```python
from build123d import *

# Parameters (mm, degrees)
SKETCH_R    = 4.3
PAD_DEPTH   = 20
FILLET_R    = 2.5
FILLET001_R = 5


with BuildPart() as part:
    # Sketch → Pad (new body)
    with BuildSketch(Plane.XY):
        with BuildLine():
            ThreePointArc((7, 0), (0, 7), (-7, 0))
            ThreePointArc((-10.818791, -6.235375), (-8.030558, -3.655922), (-7, 0))
            Line((-10.818791, -6.235375), (10.818791, -6.235375))
            ThreePointArc((7, 0), (8.030558, -3.655922), (10.818791, -6.235375))
        make_face()
        Circle(SKETCH_R, mode=Mode.SUBTRACT)
    extrude(amount=PAD_DEPTH)

    # Fillet
    fillet_edges = [part.edges().sort_by_distance(p)[0] for p in [
        (0, 7, 20),
        (8.030558, -3.655922, 20),
        (-8.030558, -3.655922, 20),
    ]]
    fillet(fillet_edges, radius=FILLET_R)

    # Fillet001
    fillet001_edges = [part.edges().sort_by_distance(p)[0] for p in [
        (0, 7, 0),
        (-8.030558, -3.655922, 0),
        (8.030558, -3.655922, 0),
    ]]
    fillet(fillet001_edges, radius=FILLET001_R)


solid = part.part
```
Check sheet for the modelled part. Datum: model origin and axes. Units: mm. Coordinates: 2 decimals unless noted, no trailing zeros. Write each loop counter-clockwise with the first axis right and the second up, starting at its lowest first coordinate (ties: lowest second). Pieces come first, ordered by that corner, then holes. Notation, with made-up numbers: (69, 49) - (107, 49) arc R11 cw to (107, 66) - close; hole circle Ø3 at (-26, 22.25). An arc over 180 degrees is marked (long way). One line per question, with ' | ' between items.
Item 1: Thickness scan on line 1 (X direction, y = 0, z = 12); line 2 (Y direction, x = 0, z = 8); line 3 (Y direction, x = 7.25, z = 2). Record the ranges inside material, lowest first. Write a range as [from, to].
Determined:
line 1: x = [-7, -4.3], [4.3, 7] | line 2: y = [-6.24, -4.3], [4.3, 7] | line 3: y = [-6.24, -4.29]
Item 2: Gauge pin test, flat ends, axial feed: P1, Ø10, axis at x = 4.5, z = 6.5, coming from the +Y side; P2, Ø1, axis at y = -4.5, z = 15.5, coming from the -X side; P3, Ø1.5, axis at y = 3, z = 3, coming from the +X side. Record the tip position at first contact, or that the pin passes through.
Determined:
P1: stops at y = 7 | P2: stops at x = -9.1 | P3: stops at x = 6.47
Item 3: Mould release check, pull along X, two halves, no side actions. Record for faces 1 (the face through (-4.296, 0.189, 9.86)), 2 (the face through (0, -5, 0)): pulls with the +X half, pulls with the -X half, needs draft (parallel to the pull), parting line crosses it, or undercut.
Determined:
face 1: undercut | face 2: needs draft
Item 4: Sectioned sample at A-A on z = 11. Record the boundary of the cut face in (x, y), plus the area to 3 significant figures.
Determined:
outline: (-10.82, -6.24) - (10.82, -6.24) arc R7 cw to (7, 0) arc R7 ccw to (-7, 0) arc R7 cw to start; hole circle Ø8.6 at (0, 0) | area: 120 mm2
